The drawing under review shows one solid part. Ordinate dimensions are in mm from its lowest x, y, z. Round coordinates to 2 decimals unless told otherwise and drop trailing zeros. Order: outer loops, then holes, each group sorted by start corner. A loop starts at its lowest first (then second) coordinate and runs counter-clockwise, first axis right, second up.
1) To check wall thickness, follow L1, parallel to Y at x = 90, z = 1.05; L2, parallel to Y at x = 90, z = 3.15; L3, parallel to Y at x = 59, z = 0.8 (1 decimal). State the ranges of each line that lie inside material, in increasing order.
2) Clearance check with flat-ended pins moving along their axes: P1, Ø3, axis at x = 87.5, y = 20.5, coming from the +Z side; P2, Ø2, axis at x = 27.5, z = 4.5, coming from the -Y side; P3, Ø1.5, axis at y = 154, z = 4.5, coming from the +X side; P4, Ø3, axis at x = 148.34, y = 148.34, coming from the +Z side. State where each tip first meets the part, or that it passes through.
3) Consider section B-B (x = 62). Give the boundary of the cut face in (y, z), then the cut area to 3 significant figures.
4) Consider section A-A (y = 115). Give the boundary of the cut face in (x, z), then the cut area to 3 significant figures.
5) Consider section C-C (z = 1.1). Give the boundary of the cut face in (x, y), then the cut area to 3 significant figures.
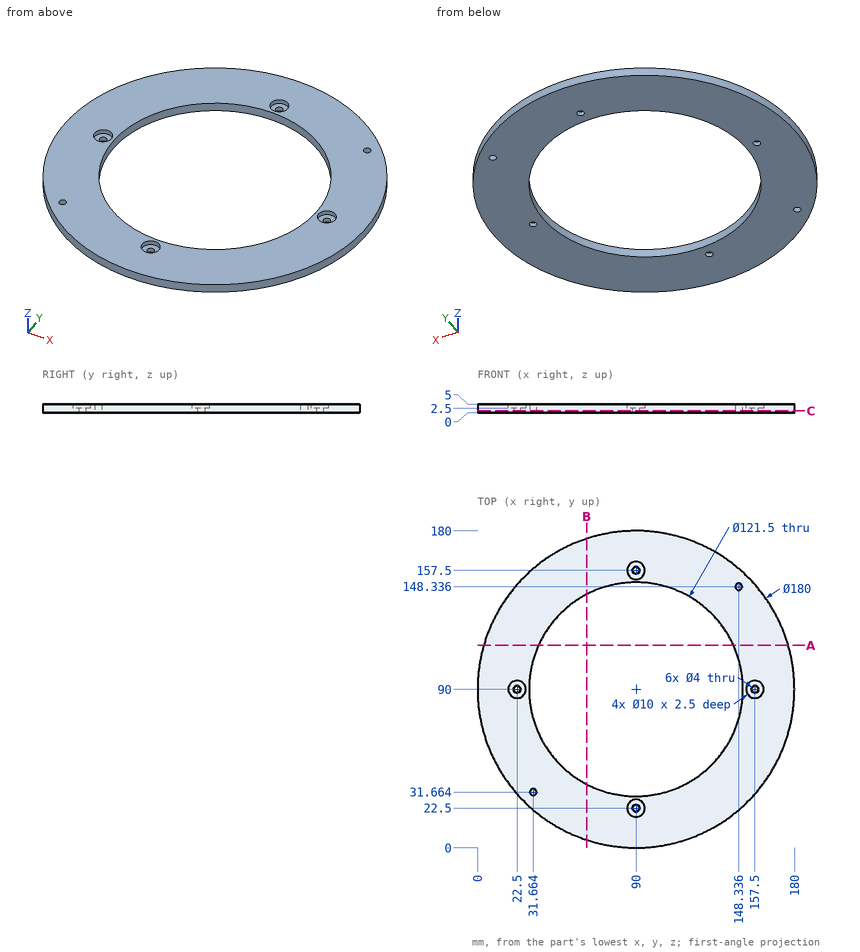
Answer below:
1. L1: y = 0 to 20.5, 24.5 to 29.25, 150.75 to 155.5, 159.5 to 180
1. L2: y = 0 to 17.5, 27.5 to 29.25, 150.75 to 152.5, 162.5 to 180
1. L3: y = 5.5 to 37.8, 142.2 to 174.5
2. P1: stops at z = 2.5
2. P2: stops at y = 24.29
2. P3: stops at x = 154.03
2. P4: passes through
3. outline: (4.47, 0) - (36.09, 0) - (36.09, 5) - (4.47, 5) - close; (143.91, 0) - (175.53, 0) - (175.53, 5) - (143.91, 5) - close
3. area: 316 mm2
4. outline: (3.54, 0) - (34.63, 0) - (34.63, 5) - (3.54, 5) - close; (145.37, 0) - (176.46, 0) - (176.46, 5) - (145.37, 5) - close
4. area: 311 mm2
5. outline: circle Ø180 at (90, 90); hole circle Ø4 at (22.5, 90); hole circle Ø121.5 at (90, 90); hole circle Ø4 at (31.66, 31.66); hole circle Ø4 at (90, 22.5); hole circle Ø4 at (90, 157.5); hole circle Ø4 at (148.34, 148.34); hole circle Ø4 at (157.5, 90)
5. area: 13,800 mm2
